Can you work these out from the model? Positions are in its coordinate system, mm. A direction names the side the tool comes from. Round coordinates to 2 decimals unless told otherwise and drop trailing zeros. Order: outer loops, then holes, each group sorted by start corner. A loop starts at its lowest first (then second) coordinate and runs counter-clockwise, first axis right, second up. Notation, with made-up numbers: M 7,-23 L 52,-23 A19 ccw 52,-6 Z; hole C 34.25,50 d5. An arc over 180 degrees is marked long. Answer as a JSON object with one key per item and string values. Group by question number.
```python
from build123d import *

# Parameters (mm, degrees)
SKETCH_1_W      = 9.55
SKETCH_1_H      = 16
EXTRUDE_1_DEPTH = 17
SKETCH_2_R      = 0.6
EXTRUDE_2_DEPTH = 4
FILLET_1_R      = 1


with BuildPart() as part:
    # 草图1 → 拉伸1 (new body)
    with BuildSketch(Plane(origin=(0, 0, 0), x_dir=(1, 0, 0), z_dir=(0, 1, 0))):
        Rectangle(SKETCH_1_W, SKETCH_1_H)
    extrude(amount=EXTRUDE_1_DEPTH)

    # 草图2 → 拉伸2 (add)
    with BuildSketch(Plane.XZ):
        with Locations(Location((-2, 0, 0), (0, 0, 90))):
            Circle(SKETCH_2_R)
    extrude(amount=EXTRUDE_2_DEPTH)

    # 圆角1
    fillet_1_edges = [part.edges().sort_by_distance(p)[0] for p in [
        (0, 17, -8),
        (0, 17, 8),
    ]]
    fillet(fillet_1_edges, radius=FILLET_1_R)


solid = part.part
```
1) If we section it at D-D on x = 0.75: Write out the boundary of the cut face in (y, z), plus the area to 3 significant figures.
2) I need wall thicknesses on line 1 along Y through (x, z) = (-3.5, 3). Which ranges of the line are inside material? Lowest first, please.
3) If we section it at C-C on y = -1.5: Write out the boundary of the cut face in (x, z), plus the area to 3 significant figures.
4) If we section it at B-B on z = 0: Write out the boundary of the cut face in (x, y) (3 decimals), plus the area to 3 significant figures.
5) If we section it at A-A on x = -2: Write out the boundary of the cut face in (y, z), plus the area to 3 significant figures.
6) Which directions (+Z, -Z, +X, -X, +Y, -Y) give clear straight access to the entire face, cutting with the end or side of a thin tool? Please do faces 1 (the face through (0, 8, 8)), 2 (the face through (-2.595, -1.972, -0.078)).
Findings:
{
 "1": {"outline": "M 0,-8 L 16,-8 A1 ccw 17,-7 L 17,7 A1 ccw 16,8 L 0,8 Z", "area": "272 mm^2"},
 "2": {"line 1": "y = 0 to 17"},
 "3": {"outline": "C -2,0 d1.2", "area": "1.13 mm^2"},
 "4": {"outline": "M -4.775,0 L -2.6,0 L -2.6,-4 L -1.4,-4 L -1.4,0 L 4.775,0 L 4.775,17 L -4.775,17 Z", "area": "167 mm^2"},
 "5": {"outline": "M -4,-0.6 L 0,-0.6 L 0,-8 L 16,-8 A1 ccw 17,-7 L 17,7 A1 ccw 16,8 L 0,8 L 0,0.6 L -4,0.6 Z", "area": "276 mm^2"},
 "6": {"face 1": "+Z, +X, -X, +Y, -Y", "face 2": "-Y"}
}
